Model file for the job. Use its own axes, mm. Give positions to 0.01 mm unless a question says otherwise; leave off trailing zeros. Order: outer loops, then holes, each group sorted by start corner. A loop starts at its lowest first (then second) coordinate and runs counter-clockwise, first axis right, second up. Notation, with made-up numbers: (29.25, 29.25) -> (50.25, 29.25) arc R22 ccw to (50.25, 66.25) -> close; hole circle Ø4 at (39, 32). An arc over 180 degrees is marked (long way). Use CSV: the item, a comma, the result in double quotes. Start each with the question number.
1. Drop flat-ended pins along their axis: pin 1 (1.5 mm diameter, centred on y = -1, z = -82.5, fed in from -X); pin 2 (0.9 mm diameter, centred on y = -2, z = -152, fed in from -X); pin 3 (6.5 mm diameter, centred on x = -48, z = -100, fed in from -Y); pin 4 (1.5 mm diameter, centred on y = -1.5, z = -83, fed in from -X). Give the stop position or say it passes through.
2. Wall check: line 1 (Z direction, x = 25, y = -2.35); line 2 (Z direction, x = 16, y = -1.5); line 3 (X direction, y = -1.6, z = -152). Give the ranges that are in metal, low to high. Write a range as from..to.
3. Cut at A-A on x = -106. List the corners of the cut face in (y, z), then the cut area to 3 significant figures.
4. Cut at B-B on y = -1.6. Give the number of separate pieces and of enclosed holes in the cut face, then the cut area to 3 significant figures.
5. Pull direction X, two halves, no side cores. Call faces 1 (the flat face through (-140, -2, -150)), 2 (the flat face through (-2, 0, -119)), 3 (the cylindrical face through (-96.437, -1.479, -109.645)): released by +X, released by -X, zero draft, split by the parting line, or undercut.
```python
from build123d import *

# Parameters (mm, degrees)
BASE_FLANGE1_START = -3
BASE_FLANGE1_DEPTH = 3
SKETCH6_R          = 1.55
CUT_EXTRUDE1_DEPTH = 10
SKETCH7_R          = 1.55
CUT_EXTRUDE2_DEPTH = 10
SKETCH8_W          = 50.2
SKETCH8_H          = 3.05
SKETCH8_W_2        = 25.1
SKETCH8_W_3        = 3.05
SKETCH8_H_2        = 15.1
CUT_EXTRUDE5_DEPTH = 10
SKETCH12_R         = 15.05
SKETCH12_R_2       = 2.05
CUT_EXTRUDE6_DEPTH = 10


# Read off the part's stored shape, not the designer's step: Base-Flange1
with BuildPart() as part:
    # Base-Flange1 outline → Base-Flange1 (new body)
    with BuildSketch(Plane(origin=(0, 0, 0), x_dir=(1, 0, 0), z_dir=(0, 1, 0)).offset(BASE_FLANGE1_START)):
        with BuildLine():
            Line((-127.928932188, 76), (127.928932188, 76))
            ThreePointArc((127.928932188, 76), (129.84234935, 76.380602337), (131.464466094, 77.464466094))
            Line((131.464466094, 77.464466094), (148.535533906, 94.535533906))
            ThreePointArc((148.535533906, 94.535533906), (149.619397663, 96.15765065), (150, 98.071067812))
            Line((150, 98.071067812), (150, 137.928932188))
            ThreePointArc((150, 137.928932188), (149.619397663, 139.84234935), (148.535533906, 141.464466094))
            Line((148.535533906, 141.464466094), (131.464466094, 158.535533906))
            ThreePointArc((131.464466094, 158.535533906), (129.84234935, 159.619397663), (127.928932188, 160))
            Line((127.928932188, 160), (-127.928932188, 160))
            ThreePointArc((-127.928932188, 160), (-129.84234935, 159.619397663), (-131.464466094, 158.535533906))
            Line((-131.464466094, 158.535533906), (-148.535533906, 141.464466094))
            ThreePointArc((-148.535533906, 141.464466094), (-149.619397663, 139.84234935), (-150, 137.928932188))
            Line((-150, 137.928932188), (-150, 98.071067812))
            ThreePointArc((-150, 98.071067812), (-149.619397663, 96.15765065), (-148.535533906, 94.535533906))
            Line((-148.535533906, 94.535533906), (-131.464466094, 77.464466094))
            ThreePointArc((-131.464466094, 77.464466094), (-129.84234935, 76.380602337), (-127.928932188, 76))
        make_face()
    extrude(amount=BASE_FLANGE1_DEPTH)

    # Sketch6 → Cut-Extrude1 (cut)
    with BuildSketch(Plane(origin=(0, 0, 0), x_dir=(1, 0, 0), z_dir=(0, 1, 0))):
        with Locations(Location((128, 146, 0), (0, 0, 270))):
            Circle(SKETCH6_R)
        with Locations(Location((-128, 146, 0), (0, 0, 90))):
            Circle(SKETCH6_R)
    extrude(amount=-CUT_EXTRUDE1_DEPTH, mode=Mode.SUBTRACT)

    # Sketch7 → Cut-Extrude2 (cut)
    with BuildSketch(Plane(origin=(0, 0, 0), x_dir=(1, 0, 0), z_dir=(0, 1, 0))):
        with Locations(Location((-128, 94, 0), (0, 0, 270))):
            Circle(SKETCH7_R)
        with Locations(Location((128, 94, 0), (0, 0, 90))):
            Circle(SKETCH7_R)
    extrude(amount=-CUT_EXTRUDE2_DEPTH, mode=Mode.SUBTRACT)

    # Sketch8 → Cut-Extrude5 (cut)
    with BuildSketch(Plane(origin=(0, 0, 0), x_dir=(1, 0, 0), z_dir=(0, 1, 0))):
        with Locations((0, 82.375)):
            Rectangle(SKETCH8_W, SKETCH8_H)
        with Locations((87.45, 82.375)):
            Rectangle(SKETCH8_W_2, SKETCH8_H)
        with Locations((136.475, 132.45)):
            Rectangle(SKETCH8_W_3, SKETCH8_H_2)
        with Locations((0, 152.025)):
            Rectangle(SKETCH8_W, SKETCH8_H)
        with Locations((87.45, 152.025)):
            Rectangle(SKETCH8_W_2, SKETCH8_H)
        with Locations((-87.45, 152.025)):
            Rectangle(SKETCH8_W_2, SKETCH8_H)
        with Locations((136.475, 101.55)):
            Rectangle(SKETCH8_W_3, SKETCH8_H_2)
        with Locations((-87.45, 82.375)):
            Rectangle(SKETCH8_W_2, SKETCH8_H)
        with Locations((-136.475, 101.55)):
            Rectangle(SKETCH8_W_3, SKETCH8_H_2)
        with Locations((-136.475, 132.45)):
            Rectangle(SKETCH8_W_3, SKETCH8_H_2)
    extrude(amount=-CUT_EXTRUDE5_DEPTH, mode=Mode.SUBTRACT)

    # Sketch12 → Cut-Extrude6 (cut)
    with BuildSketch(Plane(origin=(0, 0, 0), x_dir=(1, 0, 0), z_dir=(0, 1, 0))):
        with Locations(Location((-100.957746479, 124, 0), (0, 0, 270))):
            Circle(SKETCH12_R)
        with Locations(Location((100.957746479, 124, 0), (0, 0, 90))):
            Circle(SKETCH12_R)
        with Locations(Location((-48, 132, 0), (0, 0, 270))):
            Circle(SKETCH12_R_2)
        with Locations(Location((-48, 100, 0), (0, 0, 270))):
            Circle(SKETCH12_R_2)
        with Locations(Location((-16, 132, 0), (0, 0, 270))):
            Circle(SKETCH12_R_2)
        with Locations(Location((-16, 100, 0), (0, 0, 270))):
            Circle(SKETCH12_R_2)
        with Locations(Location((-32, 118, 0), (0, 0, 270))):
            Circle(SKETCH12_R_2)
        with Locations(Location((0, 118, 0), (0, 0, 270))):
            Circle(SKETCH12_R_2)
        with Locations(Location((-64, 118, 0), (0, 0, 270))):
            Circle(SKETCH12_R_2)
        with Locations(Location((64, 118, 0), (0, 0, 90))):
            Circle(SKETCH12_R_2)
        with Locations(Location((48, 132, 0), (0, 0, 90))):
            Circle(SKETCH12_R_2)
        with Locations(Location((48, 100, 0), (0, 0, 90))):
            Circle(SKETCH12_R_2)
        with Locations(Location((32, 118, 0), (0, 0, 90))):
            Circle(SKETCH12_R_2)
        with Locations(Location((16, 132, 0), (0, 0, 90))):
            Circle(SKETCH12_R_2)
        with Locations(Location((16, 100, 0), (0, 0, 90))):
            Circle(SKETCH12_R_2)
    extrude(amount=-CUT_EXTRUDE6_DEPTH, mode=Mode.SUBTRACT)


solid = part.part
```
Verdict:
1,pin 1,"x = -137.25"
1,pin 2,"x = -138.45"
1,pin 3,"y = -3"
1,pin 4,"x = -137.75"
2,line 1,"-160..-153.55, -150.5..-83.9, -80.85..-76"
2,line 2,"-160..-153.55, -150.5..-134.05, -129.95..-102.05, -97.95..-83.9, -80.85..-76"
2,line 3,"-138..-100, -74.9..-25.1, 25.1..74.9, 100..138"
3,outline,"(-3, -160) -> (0, -160) -> (0, -138.18) -> (-3, -138.18) -> close; (-3, -109.82) -> (0, -109.82) -> (0, -76) -> (-3, -76) -> close"
3,area,"167 mm^2"
4,separate pieces,"1"
4,enclosed holes,"29"
4,area,"22,000 mm^2"
5,face 1,"released by -X"
5,face 2,"zero draft"
5,face 3,"undercut"
